from build123d import *

# Parameters (mm, degrees)
SKETCH1_W           = 64.012274628
SKETCH1_H           = 75.085000506
BOSS_EXTRUDE1_DEPTH = 5


with BuildPart() as part:
    # Sketch1 → Boss-Extrude1 (new body)
    # profile 1 of 2: a face of its own
    with BuildSketch(Plane.XY):
        with Locations((61.398411242, 7.077500224)):
            Rectangle(SKETCH1_W, SKETCH1_H)
        with BuildLine():
            ThreePointArc((83.484398078, 2.429730903), (59.871437613, -17.479677368), (44.238109553, 9.157805497))
            ThreePointArc((44.238109553, 9.157805497), (59.81501285, 35.930775127), (83.520814038, 15.994205484))
            ThreePointArc((83.520814038, 15.994205484), (83.22114917, 12.52456978), (82.331029644, 9.157693158))
            ThreePointArc((82.331029644, 9.157693158), (83.193968093, 5.842784333), (83.484398078, 2.429730903))
        make_face(mode=Mode.SUBTRACT)
    # profile 2 of 2: a face of its own
    with BuildSketch(Plane.XY):
        with Locations((-2.613863386, 7.077500224)):
            Rectangle(SKETCH1_W, SKETCH1_H)
        with BuildLine():
            ThreePointArc((15.69984642, 2.429730903), (-7.913055331, -17.479687433), (-23.546481788, 9.157693158))
            ThreePointArc((-23.546481788, 9.157693158), (-7.969677608, 35.930764895), (15.736182375, 15.994205484))
            ThreePointArc((15.736182375, 15.994205484), (15.436527739, 12.524628574), (14.546438303, 9.157805497))
            ThreePointArc((14.546438303, 9.157805497), (15.409406369, 5.842843047), (15.69984642, 2.429730903))
        make_face(mode=Mode.SUBTRACT)
    extrude(amount=BOSS_EXTRUDE1_DEPTH)


solid = part.part
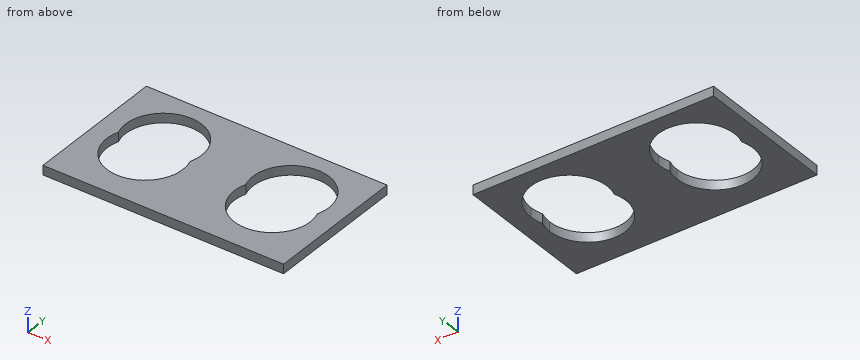
Geometry: final body of the model. Coordinates: model frame, mm. Give positions to 0.01 mm unless a question says otherwise; leave off trailing zeros. Loops run counter-clockwise (first coordinate to the right, second up) from the corner with the lowest first, then second, coordinate; pieces in that order, holes last. Notation, with made-up numbers: (81.5, 24) -> (106.5, 24) arc R20 cw to (106.5, 59) -> close; hole circle Ø2 at (20.25, 27.25). An arc over 180 degrees is marked (long way). Put each result on its own line as item: value.
1. Cut plane B-B (y = -1.5). Return the cut outline in (x, z), plus the area to 3 significant figures.
Taken from the geometry:
outline: (-34.62, 0) -> (-24.31, 0) -> (-24.31, 5) -> (-34.62, 5) -> close; (15.31, 0) -> (43.47, 0) -> (43.47, 5) -> (15.31, 5) -> close; (83.1, 0) -> (93.4, 0) -> (93.4, 5) -> (83.1, 5) -> close
area: 244 mm2
2. Cut plane A-A (x = -3). Return the cut outline in (y, z) (3 decimals).
Taken from the geometry:
outline: (-30.465, 0) -> (-17.714, 0) -> (-17.714, 5) -> (-30.465, 5) -> close; (36.175, 0) -> (44.62, 0) -> (44.62, 5) -> (36.175, 5) -> close
3. Cut plane D-D (x = 56). Return the cut outline in (y, z) (3 decimals).
Taken from the geometry:
outline: (-30.465, 0) -> (-16.411, 0) -> (-16.411, 5) -> (-30.465, 5) -> close; (34.874, 0) -> (44.62, 0) -> (44.62, 5) -> (34.874, 5) -> close
4. Cut plane C-C (z = 2.2). Return the cut outline in (x, y) (3 decimals).
Taken from the geometry:
outline: (-34.62, -30.465) -> (93.405, -30.465) -> (93.405, 44.62) -> (-34.62, 44.62) -> close; hole (-23.546, 9.158) arc R20.2 ccw (long way) to (14.546, 9.158) arc R20.236 ccw (long way) to start; hole (44.238, 9.158) arc R20.2 ccw (long way) to (82.331, 9.158) arc R20.236 ccw (long way) to start
5. Ray query, line 1 along X through (y, z) = (-14, 4.45); line 2 along X through (y, z) = (-13, 2.4); line 3 along Y through (x, z) = (62, 2.85) (3 decimals). Return the intervals inside material, ascending. Write a range as [from, to].
Taken from the geometry:
line 1: x = [-34.62, -16.25], [7.25, 51.53], [75.04, 93.4]
line 2: x = [-34.62, -17.54], [8.54, 50.25], [76.32, 93.4]
line 3: y = [-30.465, -17.729], [36.19, 44.62]
6. Pin query (flat end, axial travel): P1, Ø8, axis at x = 26, y = -12, coming from the -Z side. Return the tip coordinate at first contact, or that it passes through.
Taken from the geometry:
P1: stops at z = 0
